Build history of the part. All positions in model axes, mm. Face numbers are marked on the shaded views. A direction names the side the tool comes from. Give positions to 0.01 mm unless a question says otherwise; leave off trailing zeros. Order: outer loops, then holes, each group sorted by start corner. A loop starts at its lowest first (then second) coordinate and runs counter-clockwise, first axis right, second up. Notation, with made-up numbers: (60.25, -30.75) -> (83.25, -30.75) arc R29 cw to (83.25, 5.25) -> close; hole circle Ø5 at (-19, 74.5). An arc over 180 degrees is marked (long way). One line per item, written item: value. Start each with the question number.
(1) Pin check, flat tips, straight feed: pin 1 (8 mm diameter, centred on y = 74.5, z = 32, fed in from -X); pin 2 (12 mm diameter, centred on y = 180, z = 40, fed in from -X); pin 3 (6 mm diameter, centred on x = 25, z = 29, fed in from -Y). Stop position of each tip, or through.
(2) Saw through at A-A on x = 0. Give the cut face in (y, z) (3 decimals), plus the area to 3 significant figures.
(3) Saw through at C-C on y = 68.5. Give the cut face in (x, z) (3 decimals), plus the area to 3 significant figures.
(4) Which spindle directions (+Z, -Z, +X, -X, +Y, -Y) get a long thin tool onto all of the face, cutting with end or side? Do the marked faces 4, 5 and 6. Say none if no direction does.
(5) Saw through at D-D on y = 191. Give the cut face in (x, z).
(6) Saw through at B-B on z = 0. Give the cut face in (x, y) (3 decimals).
(7) Two-plate mould, pull along X, no slides. Class the marked faces 1, 2 and 3: +X half, -X half, draft (parallel to the pull), parting line (faces both ways), or undercut.
(8) Probe line 1 (X direction, y = 20, z = 0) (3 decimals); line 2 (Y direction, x = 11.5, z = 13); line 3 (X direction, y = 32, z = -10.5). List the from-to ranges inside material, lowest first.
```python
from build123d import *

# Parameters (mm, degrees)
SKETCH3_R          = 30.48
CUT_EXTRUDE1_DEPTH = 73.66


with BuildPart() as part:
    # Sketch1 → Revolve1 (revolve)
    with BuildSketch(Plane.XY, mode=Mode.PRIVATE) as revolve1_sk:
        Polygon((34.925, 0), (34.925, 73.66), (50.8, 73.66), (34.29, 211.836), (34.29, 228.6), (0, 228.6), (0, 0), align=None)
    revolve(revolve1_sk.sketch.rotate(Axis((0, 0, 0), (0, 1, 0)), 90), axis=Axis((0, 0, 0), (0, 1, 0)))

    # Sketch3 → Cut-Extrude1 (cut)
    with BuildSketch(Plane.XZ):
        with Locations(Location((0, 0, 0), (0, 0, 270))):
            Circle(SKETCH3_R)
    extrude(amount=-CUT_EXTRUDE1_DEPTH, mode=Mode.SUBTRACT)


solid = part.part
```
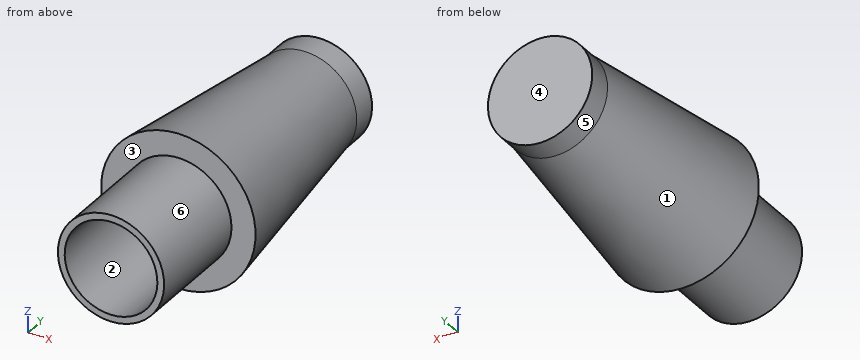
Results below:
1. pin 1: stops at x = -42.33
1. pin 2: stops at x = -17.29
1. pin 3: stops at y = 73.66
2. outline: (0, -34.925) -> (73.66, -34.925) -> (73.66, -50.8) -> (211.836, -34.29) -> (228.6, -34.29) -> (228.6, 34.29) -> (211.836, 34.29) -> (73.66, 50.8) -> (73.66, 34.925) -> (0, 34.925) -> (0, 30.48) -> (73.66, 30.48) -> (73.66, -30.48) -> (0, -30.48) -> close
2. area: 13,600 mm²
3. outline: circle Ø69.85 at (0, 0); hole circle Ø60.96 at (0, 0)
3. area: 913 mm²
4. face 4: +Z, -Z, +X, -X, +Y
4. face 5: +Y
4. face 6: -Y
5. outline: circle Ø73.56 at (0, 0)
6. outline: (-50.8, 73.66) -> (-34.925, 73.66) -> (-34.925, 0) -> (-30.48, 0) -> (-30.48, 73.66) -> (30.48, 73.66) -> (30.48, 0) -> (34.925, 0) -> (34.925, 73.66) -> (50.8, 73.66) -> (34.29, 211.836) -> (34.29, 228.6) -> (-34.29, 228.6) -> (-34.29, 211.836) -> close
7. face 1: parting line
7. face 2: undercut
7. face 3: draft
8. line 1: x = -34.925 to -30.48, 30.48 to 34.925
8. line 2: y = 73.66 to 228.6
8. line 3: x = -33.31 to -28.61, 28.61 to 33.31
